For this review, take the finished solid that the model builds, in its own axes (mm). Face numbers are marked on the shaded views. A direction names the side the tool comes from. Coordinates: 2 decimals unless noted, no trailing zeros. Loops run counter-clockwise (first coordinate to the right, second up) from the corner with the lowest first, then second, coordinate; pieces in that order, holes last.
1. Clearance check with flat-ended pins moving along their axes: P1, Ø6, axis at x = 7.5, y = 49, coming from the +Z side; P2, Ø12, axis at y = 69, z = -2, coming from the +X side; P3, Ø13.5, axis at x = 4, y = -18.5, coming from the -Z side; P4, Ø6.5, axis at x = 0, y = -16.03, coming from the +Z side. State where each tip first meets the part, or that it passes through.
2. Take a section at B-B, the plane x = 0. Count the separate pieces of the cut face and the enclosed holes in it, then the cut area to 3 significant figures.
3. Take a section at A-A, the plane y = 30. State the section outline as (x, z) points, then the cut area to 3 significant figures.
4. To check wall thickness, follow probe 1 along Y at (x, z) = (0, -4); probe 2 along Y at (x, z) = (0, 8); probe 3 along Z at (x, y) = (0.5, 45). State the ranges of each line that lie inside material, in increasing order.
5. Machinability: for the marked faces 1 and 2, which of the approach directions +Z, -Z, +X, -X, +Y, -Y give a long, thin tool a straight path to every point of the face, cutting with its end or side? Answer none if there is none.
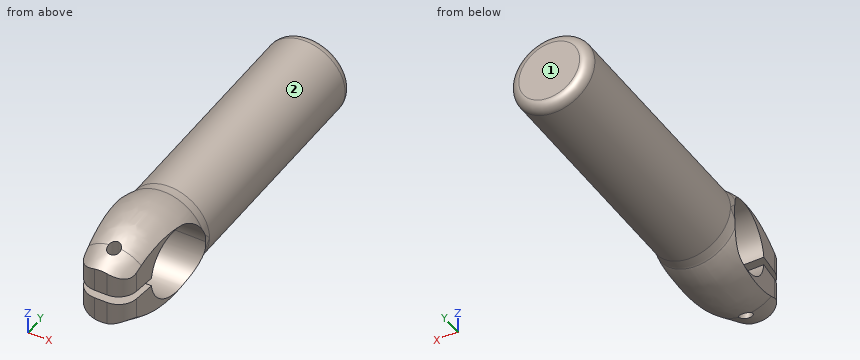
```python
from build123d import *

# Parameters (mm, degrees)
F1_DEPTH = 12.5
F3_R     = 12.5
F4_DEPTH = 74
F5_R     = 10
F8_R     = 2
F9_DEPTH = 25
F10_R    = 3


with BuildPart() as f1:
    # F0 (on Right) → F1 (new body, symmetric)
    with BuildSketch(Plane.YZ):
        with BuildLine():
            ThreePointArc((-10.9212489831, 1.3138952199), (0.6581265782, 10.9802945956), (11, 0))
            Line((11, 0), (13, 0))
            Line((13, 0), (13, 12.5))
            ThreePointArc((13, 12.5), (-1.3107386008, 15.0012988608), (-15.5343561829, 12.0445374281))
            Line((-15.5343561829, 12.0445374281), (-23.0306010843, 8.9284532397))
            Line((-23.0306010843, 8.9284532397), (-23.0306010843, 1.3138952199))
            Line((-23.0306010843, 1.3138952199), (-10.9212489831, 1.3138952199))
        make_face()
    extrude(amount=F1_DEPTH, both=True)

    # F2: F1 across plane


with BuildPart() as f1_1:
    add(f1.part)
    add(f1.part.mirror(Plane.XY))

    # F3 (on face) → F4 (join)
    with BuildSketch(Plane(origin=(0, 13, 0), x_dir=(-1, 0, 0), z_dir=(0, 1, 0))):
        Circle(F3_R)
    extrude(amount=F4_DEPTH)

    # F5
    f5_edges = [f1_1.edges().sort_by_distance(p)[0] for p in [
        (12.5, -23.030601, 5.121174),
        (-12.5, -23.030601, 5.121174),
        (-12.5, -23.030601, -5.121174),
        (12.5, -23.030601, -5.121174),
    ]]
    fillet(f5_edges, radius=F5_R)

    # F6 (on Right) → F7 (revolve, cut)
    with BuildSketch(Plane.YZ):
        with BuildLine():
            ThreePointArc((9.8683147581, 13.0030242948), (11.414086549, 12.6265569062), (13, 12.5))
            Line((13, 12.5), (46, 12.5))
            Line((46, 12.5), (46, 22.5))
            Line((46, 22.5), (-23.0306010843, 22.5))
            Line((-23.0306010843, 22.5), (-23.0306010843, 8.9284532397))
            Line((-23.0306010843, 8.9284532397), (-15.5343561829, 12.0445374281))
            ThreePointArc((-15.5343561829, 12.0445374281), (-2.9192982664, 14.8103852911), (9.8683147581, 13.0030242948))
        make_face()
    revolve(axis=Axis((0, 5.5, 0), (0, 1, 0)), mode=Mode.SUBTRACT)

    # F8 (on Top) → F9 (cut, symmetric)
    with BuildSketch(Plane.XY):
        with Locations((0, -16.0306010843)):
            Circle(F8_R)
        with BuildLine():
            Line((-7.971597998, -17.6137111518), (-9.9523894576, 2.6714647925))
            Line((-9.9523894576, 2.6714647925), (-25, 0))
            Line((-25, 0), (-25, -50))
            Line((-25, -50), (25, -50))
            Line((25, -50), (25, 0))
            Line((25, 0), (9.9523894576, 2.6714647925))
            Line((9.9523894576, 2.6714647925), (7.971597998, -17.6137111518))
            ThreePointArc((7.971597998, -17.6137111518), (6.0312119514, -21.4746229342), (2, -23.0306010843))
            Line((2, -23.0306010843), (-2, -23.0306010843))
            ThreePointArc((-2, -23.0306010843), (-6.0312119514, -21.4746229342), (-7.971597998, -17.6137111518))
        make_face()
    extrude(amount=F9_DEPTH, both=True, mode=Mode.SUBTRACT)

    # F10
    f10_edges = [f1_1.edges().sort_by_distance(p)[0] for p in [
        (12.5, 87, 0),
    ]]
    fillet(f10_edges, radius=F10_R)


solid = f1_1.part
```
Results list:
1. P1: stops at z = 11.66
1. P2: stops at x = 12.5
1. P3: stops at z = -13.15
1. P4: stops at z = 13.06
2. separate pieces: 3
2. enclosed holes: 0
2. area: 2,300 mm2
3. outline: circle Ø25 at (0, 0)
3. area: 491 mm2
4. probe 1: y = -23.03 to -18.03, -14.03 to -10.25, 10.25 to 87
4. probe 2: y = -23.03 to -18.03, -14.03 to -7.55, 7.55 to 87
4. probe 3: z = -12.49 to 12.49
5. face 1: +Z, -Z, +X, -X, +Y
5. face 2: +Y
